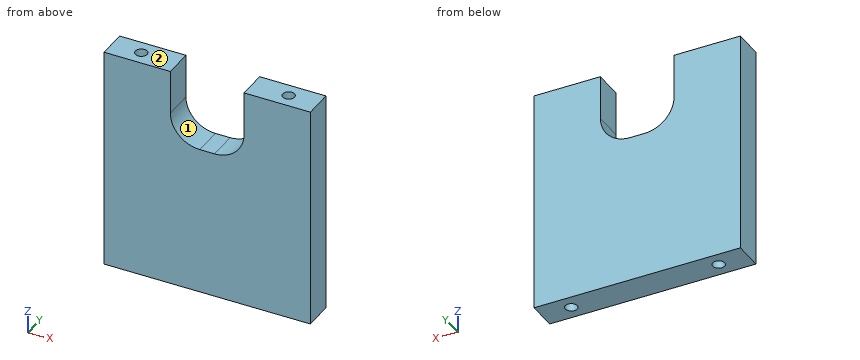
from build123d import *

# Parameters (mm, degrees)
F0_W     = 88.9
F0_H     = 12.7
F1_DEPTH = 96.6975968
F3_D     = 5.1054
F3_DEPTH = 13.97
F3_TIP   = 1.5338169022
F5_D     = 5.1054
F5_DEPTH = 13.97
F5_TIP   = 1.5338169022
F7_DEPTH = 25.4


with BuildPart() as f1:
    # F0 (on Top) → F1 (new body)
    with BuildSketch(Plane.XY):
        with Locations((-44.45, 6.35)):
            Rectangle(F0_W, F0_H)
    extrude(amount=F1_DEPTH)

    # F3
    with Locations(Plane.XY.offset(96.6975968)):
        with Locations((-76.2, 6.35), (-12.7, 6.35)):
            Hole(F3_D / 2, depth=F3_DEPTH)
            with Locations((0, 0, -(F3_DEPTH + F3_TIP / 2))):  # 118° drill point
                Cone(0, F3_D / 2, F3_TIP, mode=Mode.SUBTRACT)

    # F5
    with Locations(Plane(origin=(0, 0, 0), x_dir=(1, 0, 0), z_dir=(0, 0, -1))):
        with Locations((-76.2, -6.35), (-12.7, -6.35)):
            Hole(F5_D / 2, depth=F5_DEPTH)
            with Locations((0, 0, -(F5_DEPTH + F5_TIP / 2))):  # 118° drill point
                Cone(0, F5_D / 2, F5_TIP, mode=Mode.SUBTRACT)

    # F6 (on face) → F7 (cut)
    with BuildSketch(Plane(origin=(0, 12.7, 0), x_dir=(-1, 0, 0), z_dir=(0, 1, 0))):
        with BuildLine():
            Line((60.325, 77.6475968), (60.325, 96.6975968))
            Line((60.325, 96.6975968), (28.575, 96.6975968))
            Line((28.575, 96.6975968), (28.575, 77.6475968))
            ThreePointArc((28.575, 77.6475968), (32.2947438789, 68.6673406789), (41.275, 64.9475968))
            Line((41.275, 64.9475968), (47.625, 64.9475968))
            ThreePointArc((47.625, 64.9475968), (56.6052561211, 68.6673406789), (60.325, 77.6475968))
        make_face()
    extrude(amount=-F7_DEPTH, mode=Mode.SUBTRACT)


solid = f1.part
Geometry check sheet. Reference: the model listing, model coordinates, mm. Face numbers are marked on the shaded views. A direction names the side the tool comes from. Coordinates: 2 decimals unless noted, no trailing zeros. Order: outer loops, then holes, each group sorted by start corner. A loop starts at its lowest first (then second) coordinate and runs counter-clockwise, first axis right, second up. Notation, with made-up numbers: (-36.75, 74) -> (-27.75, 74) arc R21 cw to (-27.75, 107) -> close; hole circle Ø11 at (47.25, 12). An arc over 180 degrees is marked (long way). Use a Markdown table: item, result. Add a question column.
1. Set-up check for the marked faces 1 and 2: record each of +Z, -Z, +X, -X, +Y, -Y from which the full face is reachable in a straight line by a thin tool's end or side.
2. Cross-section at B-B (z = 12). Enter the section's corners in (x, y).
3. Cross-section at A-A (y = 11). Enter the section's corners in (x, z) (3 decimals).
4. Material ranges on L1, parallel to X at y = 6.35, z = 88 (3 decimals); L2, parallel to Y at x = -12.7, z = 89.25; L3, parallel to X at y = 9.5, z = 92 (3 decimals), recorded low to high.
5. Go/stop test with flat-tipped pins: pin 1 Ø4.5 at (x, y) = (-76.2, 6.35) entering from +Z; pin 2 Ø5 at (x, y) = (-43, 6) entering from +Z; pin 3 Ø4 at (x, y) = (-12.7, 6.35) entering from -Z. Record where each tip stops, or that it passes through.
Filled sheet:
| question | item | result |
|---|---|---|
| 1 | face 1 | +Z, +Y, -Y |
| 1 | face 2 | +Z, +X, -X, +Y, -Y |
| 2 | outline | (-88.9, 0) -> (0, 0) -> (0, 12.7) -> (-88.9, 12.7) -> close; hole circle Ø5.11 at (-76.2, 6.35); hole circle Ø5.11 at (-12.7, 6.35) |
| 3 | outline | (-88.9, 0) -> (0, 0) -> (0, 96.698) -> (-28.575, 96.698) -> (-28.575, 77.648) arc R12.7 cw to (-41.275, 64.948) -> (-47.625, 64.948) arc R12.7 cw to (-60.325, 77.648) -> (-60.325, 96.698) -> (-88.9, 96.698) -> close |
| 4 | L1 | -88.9 to -78.753, -73.647 to -60.325, -28.575 to -15.253, -10.147 to 0 |
| 4 | L2 | 0 to 3.8, 8.9 to 12.7 |
| 4 | L3 | -88.9 to -60.325, -28.575 to 0 |
| 5 | pin 1 | z = 82.55 |
| 5 | pin 2 | z = 64.97 |
| 5 | pin 3 | z = 14.3 |
